Verification items for the finished model (mm, model axes). Face numbers are marked on the shaded views. A direction names the side the tool comes from. Give positions to 0.01 mm unless a question says otherwise; leave off trailing zeros. Loops run counter-clockwise (first coordinate to the right, second up) from the corner with the lowest first, then second, coordinate; pieces in that order, holes last. Notation, with made-up numbers: (50.25, 14) - (80.25, 14) arc R32 cw to (80.25, 52) - close; hole circle Ø2 at (31, 38). An arc over 180 degrees is marked (long way). One line per question, with ' | ' between items. Start each with the question number.
1. Depth check by flat-ended pin: pin 1 Ø0.9 at (x, z) = (4.5, 78.5) entering from -Y; pin 2 Ø24 at (x, z) = (34.5, 20.5) entering from -Y. Enter the tip coordinate at first touch or a pass-through.
2. Thickness scan on line 1 along Y through (x, z) = (78, 77); line 2 along X through (y, z) = (47.5, 42.5); line 3 along X through (y, z) = (47, 61.5). Record the ranges inside material, lowest first. Write a range as from..to.
3. Section check B-B, the plane x = 60. Enter the section's corners in (y, z), then the cut area to 3 significant figures.
4. Mould release check, pull along Y, two halves, no side actions. Record for the marked faces 1 and 2: +Y half, -Y half, draft (parallel to the pull), parting line (faces both ways), or undercut.
5. Section check C-C, the plane y = 51.5. Enter the section's corners in (x, z).
6. Section check A-A, the plane y = 20. Enter the section's corners in (x, z), then the cut area to 3 significant figures.
7. Tool access check on the marked faces 3 and 4. Record the directions out of +Z, -Z, +X, -X, +Y, -Y that give a thin tool (end or side, any length) a straight path to the whole face; none if there is none.
from build123d import *

# Parameters (mm, degrees)
CYLINDER_R        = 0.8
CYLINDER_DEPTH    = 10
CYLINDER001_R     = 0.8
CYLINDER001_DEPTH = 10
CYLINDER002_R     = 0.8
CYLINDER002_DEPTH = 10
CYLINDER003_R     = 0.8
CYLINDER003_DEPTH = 10
BOX004_W          = 74
BOX004_H          = 9
BOX004_DEPTH      = 77
BOX002_W          = 74
BOX002_H          = 8
BOX002_DEPTH      = 77
BOX_W             = 80
BOX_H             = 80
BOX_DEPTH         = 80
THICKNESS_T       = 2
BOX003_W          = 80
BOX003_H          = 2
BOX003_DEPTH      = 80
CYLINDER004_W     = 6
CYLINDER004_H     = 74
CYLINDER004_ANGLE = 90
CYLINDER005_W     = 6
CYLINDER005_H     = 74
CYLINDER005_ANGLE = 90
BOX005_W          = 5
BOX005_H          = 10
BOX005_DEPTH      = 50
BOX006_W          = 5
BOX006_H          = 10
BOX006_DEPTH      = 50
BOX001_W          = 80
BOX001_H          = 2
BOX001_DEPTH      = 80


with BuildPart() as cylinder:
    # Cylinder → Cylinder (new body)
    with BuildSketch(Plane(origin=(2, 10, 70), x_dir=(1, 0, 0), z_dir=(0, 0, 1))):
        Circle(CYLINDER_R)
    extrude(amount=CYLINDER_DEPTH)


with BuildPart() as cylinder001:
    # Cylinder001 → Cylinder001 (new body)
    with BuildSketch(Plane(origin=(2, 70, 70), x_dir=(1, 0, 0), z_dir=(0, 0, 1))):
        Circle(CYLINDER001_R)
    extrude(amount=CYLINDER001_DEPTH)


with BuildPart() as cylinder002:
    # Cylinder002 → Cylinder002 (new body)
    with BuildSketch(Plane(origin=(78, 70, 70), x_dir=(1, 0, 0), z_dir=(0, 0, 1))):
        Circle(CYLINDER002_R)
    extrude(amount=CYLINDER002_DEPTH)


with BuildPart() as cylinder003:
    # Cylinder003 → Cylinder003 (new body)
    with BuildSketch(Plane(origin=(78, 10, 70), x_dir=(1, 0, 0), z_dir=(0, 0, 1))):
        Circle(CYLINDER003_R)
    extrude(amount=CYLINDER003_DEPTH)


with BuildPart() as cube004:
    # Box004 → Box004 (new body)
    with BuildSketch(Plane(origin=(3, 76, 3), x_dir=(1, 0, 0), z_dir=(0, 0, 1))):
        with Locations((37, 4.5)):
            Rectangle(BOX004_W, BOX004_H)
    extrude(amount=BOX004_DEPTH)


with BuildPart() as fusion001:
    # Box002 → Box002 (new body)
    with BuildSketch(Plane(origin=(3, -4, 3), x_dir=(1, 0, 0), z_dir=(0, 0, 1))):
        with Locations((37, 4)):
            Rectangle(BOX002_W, BOX002_H)
    extrude(amount=BOX002_DEPTH)

    # Fusion001: union Cylinder, Cylinder001, Cylinder002, Cylinder003, Cube004
    add(cylinder.part)
    add(cylinder001.part)
    add(cylinder002.part)
    add(cylinder003.part)
    add(cube004.part)


with BuildPart() as thickness:
    # Box → Box (new body)
    with BuildSketch(Plane.XY):
        with Locations((40, 40)):
            Rectangle(BOX_W, BOX_H)
    extrude(amount=BOX_DEPTH)

    # Thickness
    thickness_openings = [thickness.faces().sort_by_distance(p)[0] for p in [
        (40, 40, 80),
    ]]
    offset(amount=THICKNESS_T, openings=thickness_openings, kind=Kind.INTERSECTION)


with BuildPart() as cube003:
    # Box003 → Box003 (new body)
    with BuildSketch(Plane(origin=(0, 76, 0), x_dir=(1, 0, 0), z_dir=(0, 0, 1))):
        with Locations((40, 1)):
            Rectangle(BOX003_W, BOX003_H)
    extrude(amount=BOX003_DEPTH)


with BuildPart() as cylinder004:
    # Cylinder004 → Cylinder004 (revolve)
    with BuildSketch(Plane(origin=(0, 78, 80), x_dir=(0, 0, -1), z_dir=(-1, 0, 0))):
        with Locations((3, 37)):
            Rectangle(CYLINDER004_W, CYLINDER004_H)
    revolve(axis=Axis((0, 78, 80), (0, -1, 0)), revolution_arc=CYLINDER004_ANGLE)


with BuildPart() as cylinder005:
    # Cylinder005 → Cylinder005 (revolve)
    with BuildSketch(Plane(origin=(80, 78, 80), x_dir=(-1, 0, 0), z_dir=(0, 0, 1))):
        with Locations((3, 37)):
            Rectangle(CYLINDER005_W, CYLINDER005_H)
    revolve(axis=Axis((80, 78, 80), (0, -1, 0)), revolution_arc=CYLINDER005_ANGLE)


with BuildPart() as cube005:
    # Box005 → Box005 (new body)
    with BuildSketch(Plane(origin=(0, 43, 0), x_dir=(1, 0, 0), z_dir=(0, 0, 1))):
        with Locations((2.5, 5)):
            Rectangle(BOX005_W, BOX005_H)
    extrude(amount=BOX005_DEPTH)


with BuildPart() as cube006:
    # Box006 → Box006 (new body)
    with BuildSketch(Plane(origin=(75, 43, 0), x_dir=(1, 0, 0), z_dir=(0, 0, 1))):
        with Locations((2.5, 5)):
            Rectangle(BOX006_W, BOX006_H)
    extrude(amount=BOX006_DEPTH)


with BuildPart() as obj1:
    # Box001 → Box001 (new body)
    with BuildSketch(Plane(origin=(0, 2, 0), x_dir=(1, 0, 0), z_dir=(0, 0, 1))):
        with Locations((40, 1)):
            Rectangle(BOX001_W, BOX001_H)
    extrude(amount=BOX001_DEPTH)

    # Fusion: union Thickness, Cube003, Cylinder004, Cylinder005, Cube005, Cube006
    add(thickness.part)
    add(cube003.part)
    add(cylinder004.part)
    add(cylinder005.part)
    add(cube005.part)
    add(cube006.part)

    # Cut: cut Fusion001
    add(fusion001.part, mode=Mode.SUBTRACT)


solid = obj1.part
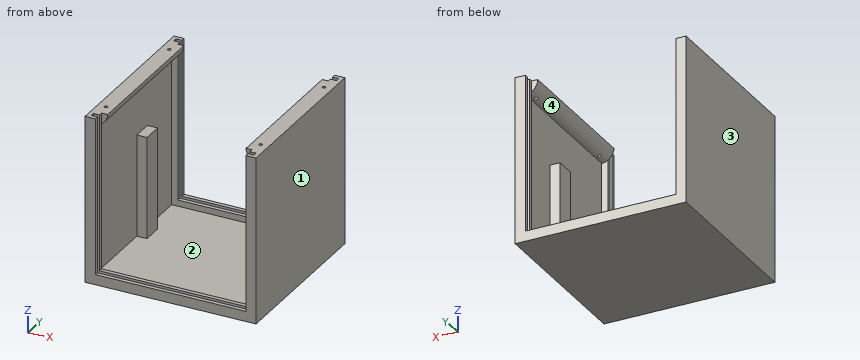
Results list:
1) pin 1: y = 4 | pin 2: through
2) line 1: -2..0, 2..9.2, 10.8..69.2, 70.8..78, 80..82 | line 2: -2..5, 75..82 | line 3: -2..0, 80..82
3) outline: (-2, -2) - (82, -2) - (82, 3) - (80, 3) - (80, 0) - (78, 0) - (78, 3) - (76, 3) - (76, 0) - (4, 0) - (4, 3) - (2, 3) - (2, 0) - (0, 0) - (0, 3) - (-2, 3) - close | area: 192 mm²
4) face 1: draft | face 2: undercut
5) outline: (-2, -2) - (82, -2) - (82, 80) - (74, 80) arc R6 ccw to (80, 74) - (80, 50) - (75, 50) - (75, 0) - (5, 0) - (5, 50) - (0, 50) - (0, 74) arc R6 ccw to (6, 80) - (-2, 80) - close
6) outline: (-2, -2) - (82, -2) - (82, 80) - (74, 80) arc R6 ccw to (80, 74) - (80, 0) - (0, 0) - (0, 74) arc R6 ccw to (6, 80) - (-2, 80) - close | area: 545 mm²
7) face 3: +Z, -Z, -X, +Y, -Y | face 4: none
